```python
from build123d import *

# Parameters (mm, degrees)
BOSS_EXTRUDE1_DEPTH = 8
SKETCH2_R           = 3
CUT_EXTRUDE1_DEPTH  = 65.249513617


with BuildPart() as part:
    # Sketch1 → Boss-Extrude1 (new, symmetric)
    with BuildSketch(Plane(origin=(0, 0, 0), x_dir=(0, 0, -1), z_dir=(1, 0, 0))):
        Polygon((0, 0), (0, -44), (-16, -44), (-16, 16), (44, 16), (44, 0), align=None)
    extrude(amount=BOSS_EXTRUDE1_DEPTH, both=True)

    # Sketch2 → Cut-Extrude1 (cut, through all)
    with BuildSketch(Plane(origin=(8, 0, 0), x_dir=(0, 0, -1), z_dir=(1, 0, 0))):
        with Locations((-8, -34)):
            Circle(SKETCH2_R)
        with Locations((-8, -14)):
            Circle(SKETCH2_R)
        with Locations((14, 8)):
            Circle(SKETCH2_R)
        with Locations((34, 8)):
            Circle(SKETCH2_R)
    extrude(amount=-CUT_EXTRUDE1_DEPTH, mode=Mode.SUBTRACT)


solid = part.part
```
Work out the finished part from the listing and answer in its coordinate system (mm). Coordinates: 2 decimals unless noted, no trailing zeros. Write each loop counter-clockwise with the first axis right and the second up, starting at its lowest first coordinate (ties: lowest second). Pieces come first, ordered by that corner, then holes. Notation, with made-up numbers: (21.5, 13) - (36.5, 13) arc R28 ccw to (36.5, 36) - close; hole circle Ø8 at (46, 11.25). An arc over 180 degrees is marked (long way). Answer as a JSON object with one key per item and string values.
Q1. Consider L1, parallel to Y at x = -4.25, z = -14; L2, parallel to Z at x = -0.5, y = 9.5; L3, parallel to Z at x = 3.75, y = -19.5. Determine where each line is inside the solid, lowest interval first. Write a range as from..to.
Results list:
{"L1": "y = 0..5, 11..16", "L2": "z = -44..-36.6, -31.4..-16.6, -11.4..16", "L3": "z = 0..16"}
Q2. For a pull along Y with two mould halves and no side action, classify faces 1 (the flat face through (0, -22, 0)), 2 (the cylindrical face through (0, 8, -31)), 3 (the flat face through (0, 0, -22)) as pulls with the +Y half, pulls with the -Y half, needs draft (parallel to the pull), parting line crosses it, or undercut.
Results list:
{"face 1": "needs draft", "face 2": "undercut", "face 3": "pulls with the -Y half"}
Q3. Find section B-B (x = -1.25). Write down the section's boundary in (y, z), plus the area to 3 significant figures.
Results list:
{"outline": "(-44, 0) - (0, 0) - (0, -44) - (16, -44) - (16, 16) - (-44, 16) - close; hole circle Ø6 at (-34, 8); hole circle Ø6 at (-14, 8); hole circle Ø6 at (8, -34); hole circle Ø6 at (8, -14)", "area": "1,550 mm^2"}
Q4. Find section D-D (y = -34). Write down the section's boundary in (x, z), plus the area to 3 significant figures.
Results list:
{"outline": "(-8, 0) - (8, 0) - (8, 5) - (-8, 5) - close; (-8, 11) - (8, 11) - (8, 16) - (-8, 16) - close", "area": "160 mm^2"}
Q5. Given pin 1 Ø4 at (x, z) = (-3.5, -4.5) entering from -Y; pin 2 Ø8 at (x, y) = (-2, -9.5) entering from -Z, each flat-ended and moving along its own axis, determine where each tip first touches the part or whether it passes through.
Results list:
{"pin 1": "stops at y = 0", "pin 2": "stops at z = 0"}
Q6. Find section A-A (z = 8). Write down the section's boundary in (x, y), plus the area to 3 significant figures.
Results list:
{"outline": "(-8, -44) - (8, -44) - (8, -37) - (-8, -37) - close; (-8, -31) - (8, -31) - (8, -17) - (-8, -17) - close; (-8, -11) - (8, -11) - (8, 16) - (-8, 16) - close", "area": "768 mm^2"}
